Autodesk Fusion 360 part; units mm, degrees
sketch "Sketch1" plane through (0, 0, 0) normal (0, 1, 0) x (1, 0, 0)
  line L0 (31, 37.5) -> (-31, 37.5)
  line L1 (-31, 37.5) -> (-31, -37.5)
  line L2 (-31, -37.5) -> (31, -37.5)
  line L3 (31, -37.5) -> (31, 37.5)
extrude "Extrude1" add sketch "Sketch1" along normal blind 34
sketch "Sketch2" plane through (0, 0, 37.5) normal (0, 0, 1) x (-1, 0, 0)
  line L0 (31, 0) -> (-31, 0)
  line L1 (-31, 0) -> (-31, -34)
  line L2 (-31, -34) -> (31, -34)
  line L3 (31, -34) -> (31, 0)
  arc A0 (19, -34) -> (-19, -34) centre (0, -34) ccw
  line L4 (19, -34) -> (-19, -34)
  dimension "d7" = 38
extrude "Extrude2" cut sketch "Sketch2" against normal blind 75 contours L2 A0 L4
sketch "Sketch3" plane through (0, 34, 0) normal (0, 1, 0) x (-1, 0, 0)
  line L0 (19, 37.5) -> (19, -37.5)
  line L1 (19, -37.5) -> (31, -37.5)
  line L2 (31, -37.5) -> (31, 37.5)
  line L3 (31, 37.5) -> (19, 37.5)
  line L4 (31, -37.5) -> (31, -31.5)
  line L5 (31, -31.5) -> (25, -31.5)
  line L6 (31, 37.5) -> (31, 31.5)
  line L7 (31, 31.5) -> (25, 31.5)
  line L8 (25, 31.5) -> (25, -31.5)
  line L9 (0.133, -37.5) -> (0.133, 37.506)
  line L10 (-30.734, -31.5) -> (-24.734, -31.5)
  line L11 (-24.734, 31.5) -> (-24.734, -31.5)
  line L12 (-30.734, 31.5) -> (-24.734, 31.5)
  dimension "d10" = 6
  dimension "d11" = 6
  dimension "d12" = 6
  dimension "d13" = 6
extrude "Extrude3" cut sketch "Sketch3" against normal blind 34 contours L2 L5 L7 L8
sketch "Sketch4" plane through (0, 34, 0) normal (0, 1, 0) x (-1, 0, 0)
  line L0 (-19, -37.5) -> (-19, 37.5)
  line L1 (-19, 37.5) -> (-31, 37.5)
  line L2 (-31, 37.5) -> (-31, -37.5)
  line L3 (-31, -37.5) -> (-19, -37.5)
  line L4 (-31, -37.5) -> (-31, -31.5)
  line L5 (-31, -31.5) -> (-25, -31.5)
  line L6 (-31, 37.5) -> (-31, 31.5)
  line L7 (-31, 31.5) -> (-25, 31.5)
  line L8 (-25, 31.5) -> (-25, -31.5)
  dimension "d16" = 6
  dimension "d17" = 6
  dimension "d18" = 6
  dimension "d19" = 6
extrude "Extrude4" cut sketch "Sketch4" against normal blind 34 contours L2 L5 L7 L8
sketch "Sketch5" plane through (25, 0, 0) normal (1, 0, 0) x (0, 1, 0)
  line L0 (34, -31.5) -> (34, 31.5)
  line L1 (34, 31.5) -> (0, 31.5)
  line L2 (0, 31.5) -> (0, -31.5)
  line L3 (0, -31.5) -> (34, -31.5)
  line L4 (0, -31.5) -> (6, -31.5)
  line L5 (6, -31.5) -> (6, 31.5)
  dimension "d22" = 6
extrude "Extrude5" cut sketch "Sketch5" against normal blind 50 contours L1 L2 L3 L4 L5
Source: CAD feature listing. Evaluate the final solid. Frame: model axes, mm. A direction names the side the tool comes from. Give positions to 0.01 mm unless a question says otherwise; leave off trailing zeros. Order: outer loops, then holes, each group sorted by start corner. A loop starts at its lowest first (then second) coordinate and runs counter-clockwise, first axis right, second up. Notation, with made-up numbers: (-40, -9) -> (12, -9) arc R3 cw to (12, -5) -> close; hole circle Ø10 at (83.25, 74). An arc over 180 degrees is marked (long way). Write item = value, one per line.
Q1. Pin query (flat end, axial travel): pin 1 (5 mm diameter, centred on x = -19.5, z = 12, fed in from -Y); pin 2 (3 mm diameter, centred on y = 25, z = 7, fed in from -X). Return the tip coordinate at first contact, or that it passes through.
Data:
pin_1 = 6
pin_2 = -25
Q2. Pull-direction query (Z, two-part tool) for faces 1 (the face through (-25, 20, 0)), 2 (the face through (0, 0, 34)), 3 (the face through (0, 13, -37.5)); classes: released by +Z, released by -Z, zero draft, split by the parting line, or undercut.
Data:
face_1 = undercut
face_2 = zero draft
face_3 = released by -Z
Q3. Cut plane C-C, the plane z = 19. Output: boundary loops of the cut face in (x, y), and give its area (3 significant figures).
Data:
outline = (-25, 6) -> (25, 6) -> (25, 34) -> (19, 34) arc R19 cw to (-19, 34) -> (-25, 34) -> close
area = 833 mm^2
Q4. Cut plane D-D, the plane x = 0. Output: boundary loops of the cut face in (y, z).
Data:
outline = (0, -37.5) -> (15, -37.5) -> (15, 37.5) -> (0, 37.5) -> (0, 31.5) -> (6, 31.5) -> (6, -31.5) -> (0, -31.5) -> close
Q5. Cut plane B-B, the plane y = 12.5. Output: boundary loops of the cut face in (x, z), and give its area (3 significant figures).
Data:
outline = (-31, -37.5) -> (31, -37.5) -> (31, -31.5) -> (25, -31.5) -> (25, 31.5) -> (31, 31.5) -> (31, 37.5) -> (-31, 37.5) -> (-31, 31.5) -> (-25, 31.5) -> (-25, -31.5) -> (-31, -31.5) -> close
area = 3,890 mm^2
Q6. Set-up query: faces 4 (the face through (0, 2, 31.5)), 5 (the face through (25, 20, 0)), 6 (the face through (24, 34, -1)), 7 (the face through (-31, 17, -35)), 8 (the face through (0, 6, 0)). Return all of +Z, -Z, +X, -X, +Y, -Y with unobstructed straight access to the full face (end or side cutting, diameter ignored); none if empty.
Data:
face_4 = -Y
face_5 = +X, +Y, -Y
face_6 = +Z, -Z, +X, -X, +Y
face_7 = +Z, -Z, -X, +Y, -Y
face_8 = +X, -X, -Y
Q7. Cut plane A-A, the plane y = 23. Output: boundary loops of the cut face in (x, z), and give its area (3 significant figures).
Data:
outline = (-31, -37.5) -> (-15.49, -37.5) -> (-15.49, 37.5) -> (-31, 37.5) -> (-31, 31.5) -> (-25, 31.5) -> (-25, -31.5) -> (-31, -31.5) -> close; (15.49, -37.5) -> (31, -37.5) -> (31, -31.5) -> (25, -31.5) -> (25, 31.5) -> (31, 31.5) -> (31, 37.5) -> (15.49, 37.5) -> close
area = 1,570 mm^2
Q8. Material intervals for line 1 (Z direction, x = -27.5, y = 5.5); line 2 (X direction, y = 31, z = 12); line 3 (X direction, y = 17, z = -24), sorted ascending. Write a range as from..to.
Data:
line_1 = -37.5..-31.5, 31.5..37.5
line_2 = -25..-18.76, 18.76..25
line_3 = -25..-8.49, 8.49..25
